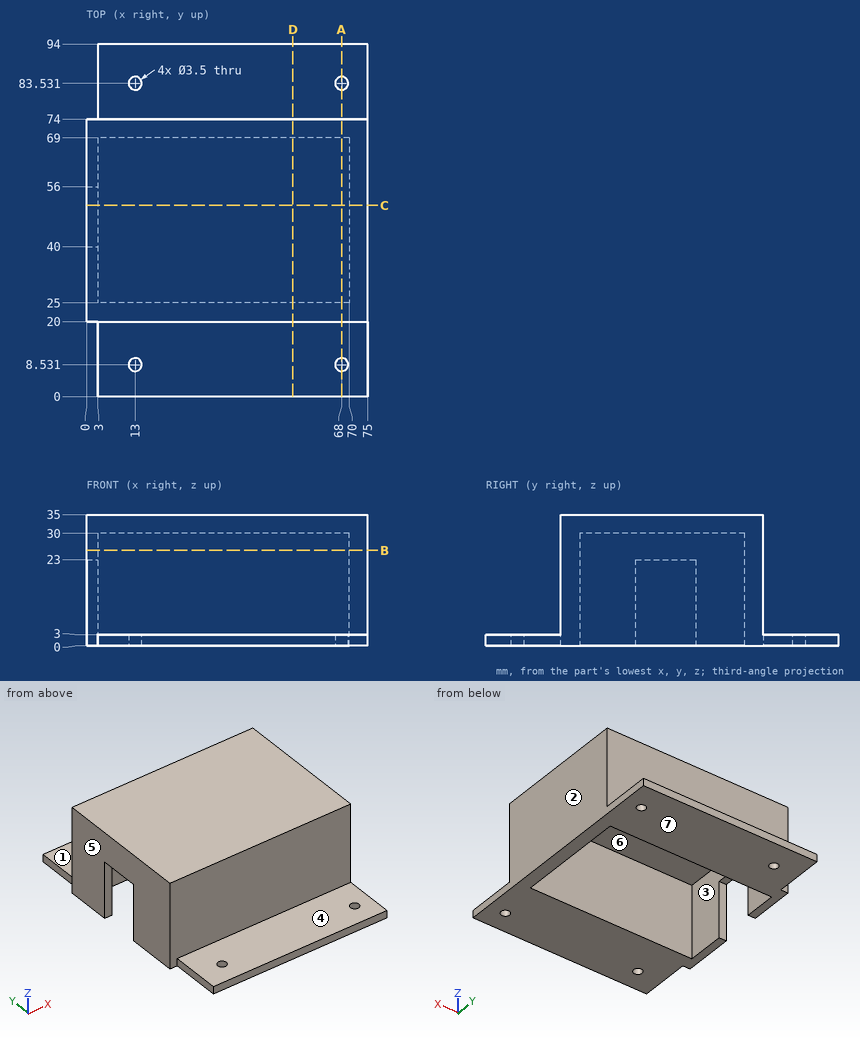
Check sheet for the drawn part. Datum: minimum x, y, z corner. Units: mm. A direction names the side the tool comes from. Give positions to 0.01 mm unless a question says otherwise; leave off trailing zeros. Write each loop counter-clockwise with the first axis right and the second up, starting at its lowest first coordinate (ties: lowest second). Pieces come first, ordered by that corner, then holes.
(1) Access from +Z, -Z, +X, -X, +Y, -Y to the whole of each face (thin tool, end or side, straight path). Record for the marked faces 1, 2, 3 and 4.
(2) Cross-section at B-B (z = 25.5). Enter the section's corners in (x, y), plus the area to 3 significant figures.
(3) Cross-section at D-D (x = 55). Enter the section's corners in (y, z).
(4) Material ranges on line 1 (Y direction, x = 68, z = 0.7); line 2 (Y direction, x = 39, z = 21); line 3 (X direction, y = 59.5, z = 6.5), recorded low to high.
(5) Cross-section at C-C (y = 51). Enter the section's corners in (x, z), plus the area to 3 significant figures.
(6) Mould release check, pull along X, two halves, no side actions. Record for the marked faces 5, 6 and 7: +X half, -X half, draft (parallel to the pull), parting line (faces both ways), or undercut.
(7) Gauge pin test, flat ends, axial feed: pin 1 (10 mm diameter, centred on x = 21.5, y = 83.5, fed in from +Z); pin 2 (10.5 mm diameter, centred on x = 31, z = 14.5, fed in from -Y); pin 3 (6 mm diameter, centred on x = 11.5, y = 65.5, fed in from -Z). Record the tip position at first contact, or that the pin passes through.
(8) Cross-section at A-A (x = 68). Enter the section's corners in (y, z), plus the area to 3 significant figures.
Worked out:
1. face 1: +Z, +X, -X, +Y
1. face 2: +Z, -Z, +X, +Y, -Y
1. face 3: -Z
1. face 4: +Z, +X, -X, -Y
2. outline: (0, 20) - (75, 20) - (75, 74) - (0, 74) - close; hole (3, 25) - (70, 25) - (70, 69) - (3, 69) - close
2. area: 1,100 mm2
3. outline: (0, 0) - (25, 0) - (25, 30) - (69, 30) - (69, 0) - (94, 0) - (94, 3) - (74, 3) - (74, 35) - (20, 35) - (20, 3) - (0, 3) - close
4. line 1: y = 0 to 6.78, 10.28 to 25, 69 to 81.78, 85.28 to 94
4. line 2: y = 20 to 25, 69 to 74
4. line 3: x = 0 to 3, 70 to 75
5. outline: (0, 23) - (3, 23) - (3, 30) - (70, 30) - (70, 0) - (75, 0) - (75, 35) - (0, 35) - close
5. area: 546 mm2
6. face 5: -X half
6. face 6: undercut
6. face 7: draft
7. pin 1: stops at z = 3
7. pin 2: stops at y = 20
7. pin 3: stops at z = 30
8. outline: (0, 0) - (6.78, 0) - (6.78, 3) - (0, 3) - close; (10.28, 0) - (25, 0) - (25, 30) - (69, 30) - (69, 0) - (81.78, 0) - (81.78, 3) - (74, 3) - (74, 35) - (20, 35) - (20, 3) - (10.28, 3) - close; (85.28, 0) - (94, 0) - (94, 3) - (85.28, 3) - close
8. area: 669 mm2
